from build123d import *

# Parameters (mm, degrees)
F0_W           = 300
F0_H           = 100
F1_DEPTH       = 5
F2_D           = 5.25
F2_CSINK_D     = 11.2
F2_CSINK_ANGLE = 90
F3_R           = 1.5


with BuildPart() as f1:
    # F0 (on Top) → F1 (new body)
    with BuildSketch(Plane.XY):
        with Locations((-150, 50)):
            Rectangle(F0_W, F0_H)
    extrude(amount=-F1_DEPTH)

    # F2 (through all)
    with Locations(Plane.XY):
        with Locations((-290, 10), (-270, 10), (-30, 10), (-10, 10), (-30, 90), (-10, 90), (-290, 90), (-270, 90)):
            CounterSinkHole(F2_D / 2, F2_CSINK_D / 2, counter_sink_angle=F2_CSINK_ANGLE)

    # F3
    f3_edges = [f1.edges().sort_by_distance(p)[0] for p in [
        (0, 0, -2.5),
        (0, 100, -2.5),
        (-300, 0, -2.5),
        (-300, 100, -2.5),
    ]]
    fillet(f3_edges, radius=F3_R)


solid = f1.part
The model under review builds one solid part; all positions refer to its coordinate system, in mm. Give positions to 0.01 mm unless a question says otherwise; leave off trailing zeros. Order: outer loops, then holes, each group sorted by start corner. A loop starts at its lowest first (then second) coordinate and runs counter-clockwise, first axis right, second up. Notation, with made-up numbers: (80, 14) -> (124, 14) arc R34 cw to (124, 50) -> close; hole circle Ø4 at (-37, 77). An arc over 180 degrees is marked (long way). Write item = value, one per line. Start each with the question number.
(1) Draft analysis for pull direction Y (two halves, no side actions). For faces 1 (the flat face through (-300, 49, -2)), 2 (the cylindrical face through (-27.92, 88.4, -4)), 3 (the flat face through (-152, 100, -2)), state which applies: +Y half, -Y half, draft (parallel to the pull), parting line (faces both ways), or undercut.
(2) Take a section at A-A (x = -30). Write out the cut boundary in (y, z) (3 decimals).
(3) Take a section at B-B (y = 90). Write out the cut boundary in (x, z) (3 decimals), plus the area to 3 significant figures.
(4) For pin 1 Ø7 at (x, y) = (-290, 90) entering from +Z; pin 2 Ø4.5 at (x, y) = (-30, 90) entering from +Z; pin 3 Ø5 at (x, y) = (-249, 47) entering from +Z; pin 4 Ø6 at (x, y) = (-270, 10) entering from +Z, all flat-tipped, find the tip position at first contact; note any pin that passes through.
(5) For L1, parallel to X at y = 10, z = -3.7 (3 decimals); L2, parallel to Y at x = -290, z = -3.35 (3 decimals); L3, parallel to X at y = 92, z = -0.9, list the stretches that pass through material, from the lowest coordinate up. Write a range as from..to.
Returned:
q1.face_1 = draft
q1.face_2 = undercut
q1.face_3 = +Y half
q2.outline = (0, -5) -> (7.375, -5) -> (7.375, -2.975) -> (4.4, 0) -> (0, 0) -> close; (12.625, -5) -> (87.375, -5) -> (87.375, -2.975) -> (84.4, 0) -> (15.6, 0) -> (12.625, -2.975) -> close; (92.625, -5) -> (100, -5) -> (100, 0) -> (95.6, 0) -> (92.625, -2.975) -> close
q3.outline = (-300, -5) -> (-292.625, -5) -> (-292.625, -2.975) -> (-295.6, 0) -> (-300, 0) -> close; (-287.375, -5) -> (-272.625, -5) -> (-272.625, -2.975) -> (-275.6, 0) -> (-284.4, 0) -> (-287.375, -2.975) -> close; (-267.375, -5) -> (-32.625, -5) -> (-32.625, -2.975) -> (-35.6, 0) -> (-264.4, 0) -> (-267.375, -2.975) -> close; (-27.375, -5) -> (-12.625, -5) -> (-12.625, -2.975) -> (-15.6, 0) -> (-24.4, 0) -> (-27.375, -2.975) -> close; (-7.375, -5) -> (0, -5) -> (0, 0) -> (-4.4, 0) -> (-7.375, -2.975) -> close
q3.area = 1,360 mm²
q4.pin_1 = -2.1
q4.pin_2 = through
q4.pin_3 = 0
q4.pin_4 = -2.6
q5.L1 = -300..-292.625, -287.375..-272.625, -267.375..-32.625, -27.375..-12.625, -7.375..0
q5.L2 = 0..7.375, 12.625..87.375, 92.625..100
q5.L3 = -300..-294.25, -285.75..-274.25, -265.75..-34.25, -25.75..-14.25, -5.75..0
